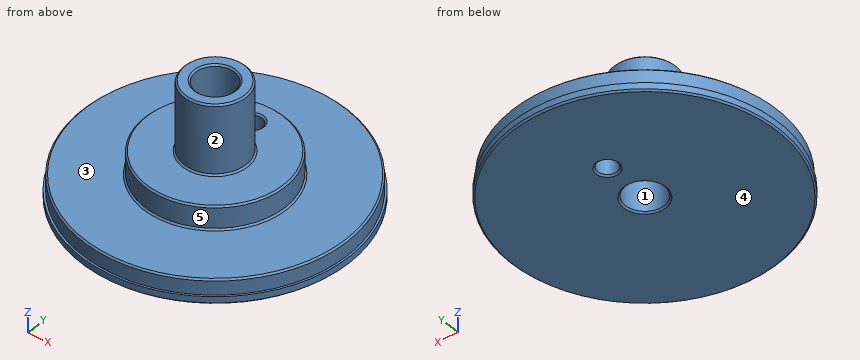
```python
from build123d import *

# Parameters (mm, degrees)
SKETCH1_R           = 17.25
SKETCH1_R_2         = 17
BOSS_EXTRUDE1_DEPTH = 1
SKETCH1_3_R         = 17
SKETCH1_3_R_2       = 9
BOSS_EXTRUDE2_DEPTH = 3
SKETCH1_4_R         = 9
SKETCH1_4_R_2       = 4
BOSS_EXTRUDE3_DEPTH = 6
SKETCH1_5_R         = 4
BOSS_EXTRUDE4_DEPTH = 15
SKETCH2_R           = 2.5
CUT_EXTRUDE1_DEPTH  = 15
SKETCH3_R           = 1.25
CUT_EXTRUDE2_DEPTH  = 6
CHAMFER1_SIZE       = 0.2


with BuildPart() as part:
    # Sketch1 → Boss-Extrude1 (new body)
    with BuildSketch(Plane.XY):
        Circle(SKETCH1_R)
        Circle(SKETCH1_R_2, mode=Mode.SUBTRACT)
    extrude(amount=BOSS_EXTRUDE1_DEPTH)

    # Sketch1<3> → Boss-Extrude2 (add)
    with BuildSketch(Plane.XY):
        Circle(SKETCH1_3_R)
        Circle(SKETCH1_3_R_2, mode=Mode.SUBTRACT)
    extrude(amount=BOSS_EXTRUDE2_DEPTH)

    # Sketch1<4> → Boss-Extrude3 (add)
    with BuildSketch(Plane.XY):
        Circle(SKETCH1_4_R)
        Circle(SKETCH1_4_R_2, mode=Mode.SUBTRACT)
    extrude(amount=BOSS_EXTRUDE3_DEPTH)

    # Sketch1<5> → Boss-Extrude4 (add)
    with BuildSketch(Plane.XY):
        Circle(SKETCH1_5_R)
    extrude(amount=BOSS_EXTRUDE4_DEPTH)

    # Sketch2 → Cut-Extrude1 (cut)
    with BuildSketch(Plane.XY.offset(15)):
        Circle(SKETCH2_R)
    extrude(amount=-CUT_EXTRUDE1_DEPTH, mode=Mode.SUBTRACT)

    # Sketch3 → Cut-Extrude2 (cut)
    with BuildSketch(Plane.XY.offset(6)):
        with Locations((0, 6)):
            Circle(SKETCH3_R)
    extrude(amount=-CUT_EXTRUDE2_DEPTH, mode=Mode.SUBTRACT)

    # Chamfer1
    chamfer1_edges = [part.edges().sort_by_distance(p)[0] for p in [
        (-4, 0, 6),
        (-9, 0, 6),
        (-4, 0, 15),
        (-2.5, 0, 15),
        (-2.5, 0, 0),
        (-1.25, 6, 0),
        (-1.25, 6, 6),
        (-17.25, 0, 0),
        (-9, 0, 3),
        (-17, 0, 3),
    ]]
    chamfer(chamfer1_edges, length=CHAMFER1_SIZE)


solid = part.part
```
The model under review builds one solid part; all positions refer to its coordinate system, in mm. Face numbers are marked on the shaded views. A direction names the side the tool comes from. Give positions to 0.01 mm unless a question says otherwise; leave off trailing zeros. Write each loop counter-clockwise with the first axis right and the second up, starting at its lowest first coordinate (ties: lowest second). Pieces come first, ordered by that corner, then holes. Notation, with made-up numbers: (-16, -29) - (22, -29) arc R23 ccw to (22, -20) - close; hole circle Ø8 at (5.25, -11). An arc over 180 degrees is marked (long way). Answer in a Markdown table with one row per item. Add a question column.
1. We need section A-A on x = 0. State how many separate pieces and enclosed holes the cut face has, then the cut area to 3 significant figures.
2. We need section C-C on z = 1.5. Write out the cut boundary in (x, y), then the cut area to 3 significant figures.
3. Insertion check: P1, Ø1, axis at x = -5.5, z = 3, coming from the -Y side; P2, Ø10, axis at x = -12, y = -6, coming from the +Z side; P3, Ø8, axis at x = 11, z = 1.5, coming from the -Y side. Each pin has a flat end and moves straight along its axis. Give the tip position at first contact, or say it passes through.
4. Tool access review of the marked faces 4 and 5: name each direction out of +Z, -Z, +X, -X, +Y, -Y from which nothing blocks a thin tool from reaching the whole face with its end or side.
5. Wall thickness on line 1 along Y through (x, z) = (0, 7.5); line 2 along X through (y, z) = (7, 4); line 3 along Z through (x, y) = (10, 12.5): over which ranges is each line inside the solid? List them lowest first. Write a range as [from, to].
6. Draft analysis for pull direction X (two halves, no side actions). For the marked faces 1, 2 and 3, state which applies: +X half, -X half, draft (parallel to the pull), parting line (faces both ways), or undercut.
7. We need section B-B on z = 13.5. Write out the cut boundary in (x, y).
Ans:
| question | item | result |
|---|---|---|
| 1 | separate pieces | 3 |
| 1 | enclosed holes | 0 |
| 1 | area | 138 mm^2 |
| 2 | outline | circle Ø34 at (0, 0); hole circle Ø5 at (0, 0); hole circle Ø2.5 at (0, 6) |
| 2 | area | 883 mm^2 |
| 3 | P1 | stops at y = -16.24 |
| 3 | P2 | stops at z = 6 |
| 3 | P3 | stops at y = -15.75 |
| 4 | face 4 | -Z, +X, -X, +Y, -Y |
| 4 | face 5 | +Z |
| 5 | line 1 | y = [-4, -2.5], [2.5, 4] |
| 5 | line 2 | x = [-5.66, -0.75], [0.75, 5.66] |
| 5 | line 3 | z = [0, 3] |
| 6 | face 1 | undercut |
| 6 | face 2 | parting line |
| 6 | face 3 | draft |
| 7 | outline | circle Ø8 at (0, 0); hole circle Ø5 at (0, 0) |
